The listing builds one solid part. Answer for the finished solid, in the listing's coordinates (mm). Face numbers are marked on the shaded views. A direction names the side the tool comes from. Coordinates: 2 decimals unless noted, no trailing zeros. Order: outer loops, then holes, each group sorted by start corner. A loop starts at its lowest first (then second) coordinate and runs counter-clockwise, first axis right, second up. Notation, with made-up numbers: (30, 64) - (64, 64) arc R22 ccw to (64, 79) - close; hole circle Ø1 at (25, 56). An arc over 180 degrees is marked (long way). Use a Markdown table: item, result. Add a question column.
Item 1: The part is cut by section B-B, the plane x = -62.5. Give the vertices of the cut face in (y, z).
Item 2: The part is cut by section D-D, the plane y = 69. Give the vertices of the cut face in (x, z).
Item 3: Find the intervals of material crossed by line 1 along Y through (x, z) = (62, 0); line 2 along Y through (x, z) = (24.5, -46.5); line 3 along X through (y, z) = (-2.5, 0), in increasing order.
Item 4: The part is cut by section C-C, the plane x = 0. Give the vertices of the cut face in (y, z).
Item 5: Flat-ended cylindrical pins translate along their axes: P1, Ø5, axis at x = 13, z = -33, coming from the +Y side; P2, Ø10, axis at x = 44, y = -0.5, coming from the +Z side; P3, Ø16, axis at x = 61, y = 1, coming from the -Z side. Find the tip coordinate at first contact, or state that the pin passes through.
Item 6: For the marked faces 4 and 5, determine the directions among +Z, -Z, +X, -X, +Y, -Y from which every point of the face is accessible in a straight line to the end or side of a thin tool.
Item 7: The mould has two halves that part along X. Classify the marked faces 1, 2 and 3: released by +X, released by -X, zero draft, split by the parting line, or undercut.
Item 8: The part is cut by section A-A, the plane z = -33.5. Give the vertices of the cut face in (x, y), then the cut area to 3 significant figures.
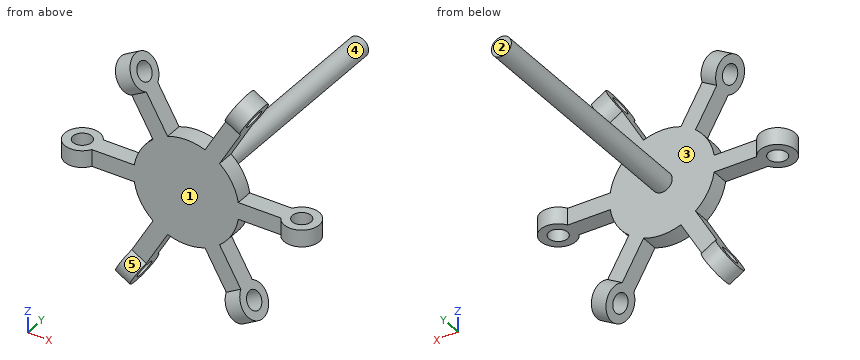
from build123d import *

# Parameters (mm, degrees)
SKETCH_1_R               = 30
EXTRUDE_1_DEPTH          = 5
SKETCH_2_W               = 50
SKETCH_2_H               = 9.6
EXTRUDE_2_DEPTH          = 5
SKETCH_3_R               = 10
EXTRUDE_3_DEPTH          = 9.6
SKETCH_4_R               = 5.3
CUT_EXTRUDE_1_DEPTH      = 10
PATTERN_CIRCULAR_1_COUNT = 6
SKETCH_5_R               = 5.7
EXTRUDE_11_4_140_DEPTH   = 140


with BuildPart() as part:
    # 草图1 → 凸台-拉伸1 (new, symmetric)
    with BuildSketch(Plane(origin=(0, 0, 0), x_dir=(1, 0, 0), z_dir=(0, 1, 0))):
        with Locations(Location((0, 0, 0), (0, 0, 270))):
            Circle(SKETCH_1_R)
    extrude(amount=EXTRUDE_1_DEPTH, both=True)

    # 草图2 → 凸台-拉伸2 (add, symmetric)
    with BuildSketch(Plane(origin=(0, 0, 0), x_dir=(1, 0, 0), z_dir=(0, 1, 0))):
        with Locations((45, 0)):
            Rectangle(SKETCH_2_W, SKETCH_2_H)
    extrude_2 = extrude(amount=EXTRUDE_2_DEPTH, both=True)

    # 草图3 → 凸台-拉伸3 (add)
    with BuildSketch(Plane.XY.offset(4.8)):
        with Locations((62.5, 0)):
            Circle(SKETCH_3_R)
    extrude_3 = extrude(amount=-EXTRUDE_3_DEPTH)

    # 草图4 → 切除-拉伸1 (cut)
    with BuildSketch(Plane.XY.offset(4.8)):
        with Locations((62.5, 0)):
            Circle(SKETCH_4_R)
    cut_extrude_1 = extrude(amount=-CUT_EXTRUDE_1_DEPTH, mode=Mode.SUBTRACT)

    # 阵列(圆周)1: 凸台-拉伸2, 凸台-拉伸3, 切除-拉伸1 ×6 about axis
    pattern_circular_1_axis = Axis((0, 5, 0), (0, -1, 0))
    add([extrude_2.rotate(pattern_circular_1_axis, i * 360 / PATTERN_CIRCULAR_1_COUNT) for i in range(1, PATTERN_CIRCULAR_1_COUNT)])
    add([extrude_3.rotate(pattern_circular_1_axis, i * 360 / PATTERN_CIRCULAR_1_COUNT) for i in range(1, PATTERN_CIRCULAR_1_COUNT)])
    add([cut_extrude_1.rotate(pattern_circular_1_axis, i * 360 / PATTERN_CIRCULAR_1_COUNT) for i in range(1, PATTERN_CIRCULAR_1_COUNT)], mode=Mode.SUBTRACT)

    # 草图5 → 细杆_直径11.4_长度140 (add)
    with BuildSketch(Plane(origin=(0, 5, 0), x_dir=(1, 0, 0), z_dir=(0, 1, 0))):
        with Locations(Location((0, 0, 0), (0, 0, 270))):
            Circle(SKETCH_5_R)
    extrude(amount=EXTRUDE_11_4_140_DEPTH)


solid = part.part
Solution:
| question | item | result |
|---|---|---|
| 1 | outline | (-10, -4.8) - (-5.3, -4.8) - (-5.3, 4.8) - (-10, 4.8) - close; (5.3, -4.8) - (10, -4.8) - (10, 4.8) - (5.3, 4.8) - close |
| 2 | outline | circle Ø11.4 at (0, 0) |
| 3 | line 1 | y = -9.99 to -5.28, 5.28 to 9.99 |
| 3 | line 2 | y = -5 to 5 |
| 3 | line 3 | x = -72.18 to -67.17, -57.83 to 57.83, 67.17 to 72.18 |
| 4 | outline | (-5, -30) - (5, -30) - (5, -5.7) - (145, -5.7) - (145, 5.7) - (5, 5.7) - (5, 30) - (-5, 30) - close |
| 5 | P1 | stops at y = 5 |
| 5 | P2 | stops at z = 61.19 |
| 5 | P3 | stops at z = -4.8 |
| 6 | face 4 | +Y |
| 6 | face 5 | none |
| 7 | face 1 | undercut |
| 7 | face 2 | zero draft |
| 7 | face 3 | undercut |
| 8 | outline | (-24.88, -5) - (-13.8, -5) - (-13.8, 5) - (-24.88, 5) - close; (13.8, -5) - (24.88, -5) - (24.88, 5) - (13.8, 5) - close |
| 8 | area | 222 mm2 |
